Can you work these out from the model? Positions are in its coordinate system, mm. Face numbers are marked on the shaded views. A direction names the side the tool comes from. Give positions to 0.01 mm unless a question says otherwise; leave off trailing zeros. Loops run counter-clockwise (first coordinate to the right, second up) from the corner with the lowest first, then second, coordinate; pieces in that order, holes last. Notation, with made-up numbers: (70, 51.25) - (81, 51.25) arc R22 ccw to (81, 88.25) - close; hole circle Ø10 at (86, 64). An arc over 180 degrees is marked (long way). Answer as a JSON object with one key per item and string values.
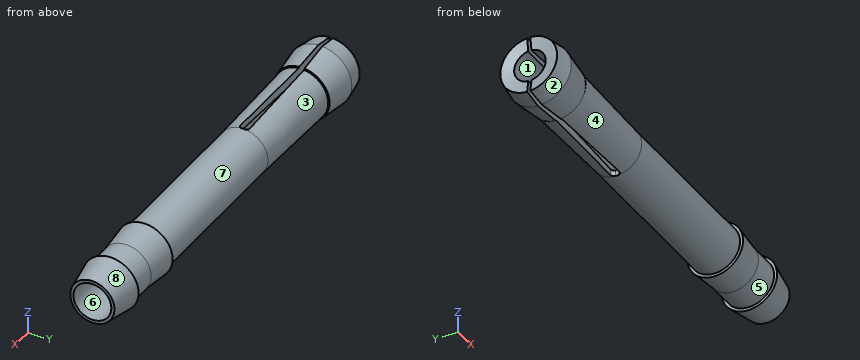
```python
from build123d import *

# Parameters (mm, degrees)
CORTE_EXTRUS_O1_DEPTH = 5


with BuildPart() as part:
    # Esboço1 → Revolução1 (revolve)
    with BuildSketch(Plane.XY, mode=Mode.PRIVATE) as revolu_o1_sk:
        Polygon((0.133333333, 1), (0, 1.8), (1.2, 2), (3.2, 1.756376953), (3.256376953, 1.7), (9.6, 1.575), (20.3, 1.575), (20.3, 1.765), (22.3, 1.575), (24, 1.575), (24, 1.765), (26, 1.4), (26, 1.2), (9.6, 1.2), align=None)
    revolve(revolu_o1_sk.sketch.rotate(Axis((0, 0, 0), (1, 0, 0)), 90), axis=Axis((0, 0, 0), (1, 0, 0)))

    # Esboço2 → Corte-extrusão1 (cut, symmetric)
    with BuildSketch(Plane.XY):
        with BuildLine():
            Line((0, 0.1), (9.395834237, 0.295746547))
            ThreePointArc((9.395834237, 0.295746547), (9.539940787, 0.238676521), (9.6, 0.095789935))
            Line((9.6, 0.095789935), (9.6, -0.095789935))
            ThreePointArc((9.6, -0.095789935), (9.539940787, -0.238676521), (9.395834237, -0.295746547))
            Line((9.395834237, -0.295746547), (0, -0.1))
            Line((0, -0.1), (0, 0.1))
        make_face()
    extrude(amount=CORTE_EXTRUS_O1_DEPTH, both=True, mode=Mode.SUBTRACT)


solid = part.part
```
1) I'm going to push flat-ended pins straight in: P1, Ø1.4, axis at y = 0, z = 0, coming from the +X side; P2, Ø1, axis at x = 8, z = -0.5, coming from the -Y side; P3, Ø1.1, axis at y = -0.5, z = -0.5, coming from the -X side; P4, Ø1.5, axis at x = 19.5, z = -1.5, coming from the -Y side. Where does each tip first touch, or does it pass through?
Check sheet entries:
{"P1": "through", "P2": "y = -1.61", "P3": "x = 0.09", "P4": "y = -1.38"}
2) Which directions (+Z, -Z, +X, -X, +Y, -Y) give clear straight access to the entire face, cutting with the end or side of a thin tool? Please do the marked faces 1, 2, 3, 4 and 5.
Check sheet entries:
{"face 1": "+X", "face 2": "-X, -Y", "face 3": "+Y", "face 4": "-Y", "face 5": "none"}
3) Imagine slicing it at B-B on x = 18. Write out the boundary of the cut face in (y, z) (3 decimals), and give its area (3 significant figures).
Check sheet entries:
{"outline": "circle Ø3.15 at (0, 0); hole circle Ø2.4 at (0, 0)", "area": "3.27 mm2"}
4) I need wall thicknesses on L1, parallel to Y at x = 16, z = 0 (3 decimals); L2, parallel to Z at x = 19.75, y = -1.05; L3, parallel to Y at x = 20.25, z = 0.3. Which ranges of each line are inside material? Lowest first, please.
Check sheet entries:
{"L1": "-1.575 to -1.2, 1.2 to 1.575", "L2": "-1.17 to -0.58, 0.58 to 1.17", "L3": "-1.55 to -1.16, 1.16 to 1.55"}
5) If we mould it in two halves opening along X, with no side actions, what happens to the marked faces 6, 7 and 8? For each: released by +X, released by -X, zero draft, split by the parting line, or undercut.
Check sheet entries:
{"face 6": "zero draft", "face 7": "undercut", "face 8": "released by +X"}
6) Imagine slicing it at A-A on x = 3.75. Write out the boundary of the cut face in (y, z).
Check sheet entries:
{"outline": "(-0.18, -1.68) - (-0.18, -1.06) arc R1.08 cw to (-0.18, 1.06) - (-0.18, 1.68) arc R1.69 ccw to start; (0.18, -1.68) arc R1.69 ccw to (0.18, 1.68) - (0.18, 1.06) arc R1.08 cw to (0.18, -1.06) - close"}
